Verification items for this drawing (mm, ordinates from the low corner). A direction names the side the tool comes from. Give positions to 0.01 mm unless a question says otherwise; leave off trailing zeros. Order: outer loops, then holes, each group sorted by start corner. A loop starts at its lowest first (then second) coordinate and runs counter-clockwise, first axis right, second up. Notation, with made-up numbers: M -1.75,73.25 L 49.25,73.25 A12 cw 49.25,89.25 Z; hole C 86,73.25 d8. An arc over 180 degrees is marked long. Answer as a JSON object with one key per item and string values.
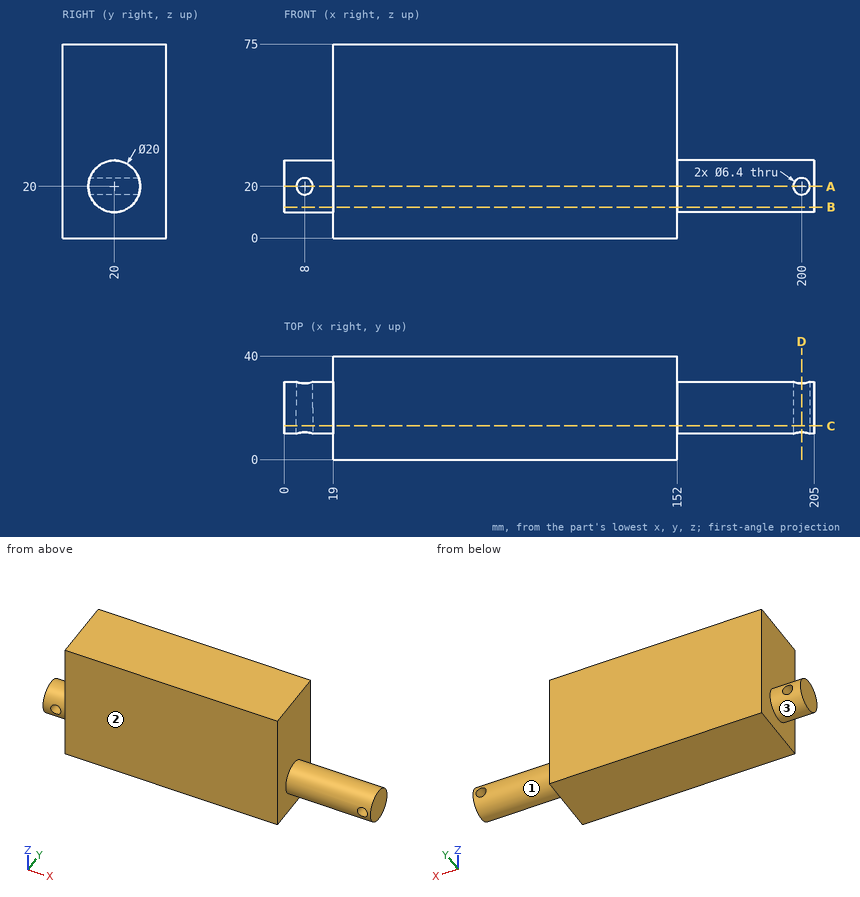
Q1. Section check C-C on y = 13. Record the cut outline in (x, z), then the cut area to 3 significant figures.
Resolved:
{"outline": "M 0,12.86 L 19,12.86 L 19,0 L 152,0 L 152,12.86 L 205,12.86 L 205,27.14 L 152,27.14 L 152,75 L 19,75 L 19,27.14 L 0,27.14 Z; hole C 8,20 d6.4; hole C 200,20 d6.4", "area": "10,900 mm²"}
Q2. Gauge pin test, flat ends, axial feed: pin 1 Ø10 at (x, y) = (35, 11) entering from -Z; pin 2 Ø7.5 at (x, z) = (200, 20) entering from -Y; pin 3 Ø8.5 at (x, z) = (8, 20) entering from +Y; pin 4 Ø10 at (y, z) = (5.5, 53.5) entering from +X. Record the tip position at first contact, or that the pin passes through.
Resolved:
{"pin 1": "stops at z = 0", "pin 2": "stops at y = 10", "pin 3": "stops at y = 30", "pin 4": "stops at x = 152"}
Q3. Tool access check on the marked faces 1, 2 and 3. Record the directions out of +Z, -Z, +X, -X, +Y, -Y that give a thin tool (end or side, any length) a straight path to the whole face; none if there is none.
Resolved:
{"face 1": "+X", "face 2": "+Z, -Z, +X, -X, -Y", "face 3": "-X"}
Q4. Section check D-D on x = 200. Record the cut outline in (y, z), then the cut area to 3 significant figures.
Resolved:
{"outline": "M 10.53,16.8 A10 ccw 29.47,16.8 Z; M 10.53,23.2 L 29.47,23.2 A10 ccw Z", "area": "188 mm²"}
Q5. Material ranges on L1, parallel to X at y = 25, z = 20; L2, parallel to X at y = 12.5, z = 7; L3, parallel to X at y = 13, z = 18, recorded low to high.
Resolved:
{"L1": "x = 0 to 4.8, 11.2 to 196.8, 203.2 to 205", "L2": "x = 19 to 152", "L3": "x = 0 to 5.5, 10.5 to 197.5, 202.5 to 205"}
Q6. Section check A-A on z = 20. Record the cut outline in (x, y).
Resolved:
{"outline": "M 0,10 L 4.8,10 L 4.8,30 L 0,30 Z; M 11.2,10 L 19,10 L 19,0 L 152,0 L 152,10 L 196.8,10 L 196.8,30 L 152,30 L 152,40 L 19,40 L 19,30 L 11.2,30 Z; M 203.2,10 L 205,10 L 205,30 L 203.2,30 Z"}
Q7. Section check B-B on z = 12. Record the cut outline in (x, y).
Resolved:
{"outline": "M 0,14 L 19,14 L 19,0 L 152,0 L 152,14 L 205,14 L 205,26 L 152,26 L 152,40 L 19,40 L 19,26 L 0,26 Z"}
